Read the model definition and answer for the solid it produces. Units are mm, in the model's axes. Give positions to 0.01 mm unless a question says otherwise; leave off trailing zeros. Loops run counter-clockwise (first coordinate to the right, second up) from the corner with the lowest first, then second, coordinate; pieces in that order, holes last. Notation, with made-up numbers: (41, 1) -> (68, 1) arc R25 ccw to (68, 40) -> close; hole circle Ø1 at (38.25, -29.75). An arc over 180 degrees is marked (long way). Write each question's results on one line, items separated by ' | '. Start each with the question number.
Item 1: Section B-B on y = 24 is taken. Write down the section's boundary in (x, z).
Item 2: Section A-A on x = 7 is taken. Write down the section's boundary in (y, z).
Item 3: Section C-C on z = 1.05 is taken. Write down the section's boundary in (x, y), and give its area (3 significant figures).
Item 4: Section D-D on x = 68 is taken. Write down the section's boundary in (y, z).
Item 5: Find the intervals of material crossed by line 1 (Y direction, x = 73.3, z = 0.9); line 2 (Y direction, x = 4, z = 0.75); line 3 (X direction, y = 47, z = 1.3), in increasing order.
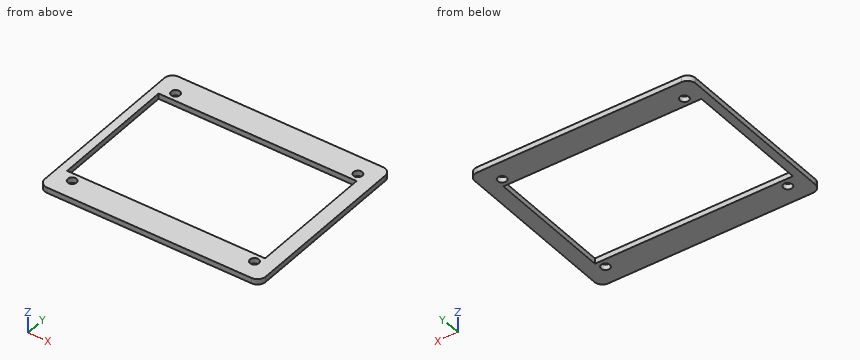
```python
from build123d import *

# Parameters (mm, degrees)
SKETCH1_W                  = 80.3
SKETCH1_H                  = 66
BOSS_EXTRUDE1_DEPTH        = 2
F_3_2_3_2_DIAMETER_HOLE1_D = 3.2
FILLET1_R                  = 3
SKETCH4_W                  = 72
SKETCH4_H                  = 46
CUT_EXTRUDE1_DEPTH         = 3


with BuildPart() as part:
    # Sketch1 → Boss-Extrude1 (new body)
    with BuildSketch(Plane.XY):
        with Locations((40.15, 33)):
            Rectangle(SKETCH1_W, SKETCH1_H)
    extrude(amount=BOSS_EXTRUDE1_DEPTH)

    # Ø3.2 (3.2) Diameter Hole1 (through all)
    with Locations(Plane.XY.offset(2)):
        with Locations((7, 59), (73.3, 59), (73.3, 7), (7, 7)):
            Hole(F_3_2_3_2_DIAMETER_HOLE1_D / 2)

    # Fillet1
    fillet1_edges = [part.edges().sort_by_distance(p)[0] for p in [
        (0, 66, 1),
        (80.3, 66, 1),
        (80.3, 0, 1),
        (0, 0, 1),
    ]]
    fillet(fillet1_edges, radius=FILLET1_R)

    # Sketch4 → Cut-Extrude1 (cut, through all)
    with BuildSketch(Plane.XY.offset(2)):
        with Locations((39, 33)):
            Rectangle(SKETCH4_W, SKETCH4_H)
    extrude(amount=-CUT_EXTRUDE1_DEPTH, mode=Mode.SUBTRACT)


solid = part.part
```
Findings:
1) outline: (0, 0) -> (3, 0) -> (3, 2) -> (0, 2) -> close; (75, 0) -> (80.3, 0) -> (80.3, 2) -> (75, 2) -> close
2) outline: (0, 0) -> (5.4, 0) -> (5.4, 2) -> (0, 2) -> close; (8.6, 0) -> (10, 0) -> (10, 2) -> (8.6, 2) -> close; (56, 0) -> (57.4, 0) -> (57.4, 2) -> (56, 2) -> close; (60.6, 0) -> (66, 0) -> (66, 2) -> (60.6, 2) -> close
3) outline: (0, 3) arc R3 ccw to (3, 0) -> (77.3, 0) arc R3 ccw to (80.3, 3) -> (80.3, 63) arc R3 ccw to (77.3, 66) -> (3, 66) arc R3 ccw to (0, 63) -> close; hole (3, 10) -> (75, 10) -> (75, 56) -> (3, 56) -> close; hole circle Ø3.2 at (7, 7); hole circle Ø3.2 at (7, 59); hole circle Ø3.2 at (73.3, 7); hole circle Ø3.2 at (73.3, 59) | area: 1,950 mm2
4) outline: (0, 0) -> (10, 0) -> (10, 2) -> (0, 2) -> close; (56, 0) -> (66, 0) -> (66, 2) -> (56, 2) -> close
5) line 1: 0 to 5.4, 8.6 to 10, 56 to 57.4, 60.6 to 66 | line 2: 0 to 10, 56 to 66 | line 3: 0 to 3, 75 to 80.3
